Geometry check sheet. Reference: the model listing, model coordinates, mm. A direction names the side the tool comes from. Coordinates: 2 decimals unless noted, no trailing zeros. Write each loop counter-clockwise with the first axis right and the second up, starting at its lowest first coordinate (ties: lowest second). Pieces come first, ordered by that corner, then holes. Notation, with made-up numbers: (56, 15) -> (69, 15) arc R14 cw to (69, 35) -> close; hole circle Ø4 at (24, 22). An arc over 180 degrees is marked (long way). Answer in a Markdown table with one row per item. Add a question column.
1. Cross-section at D-D on z = 7.5. Record the cut outline in (x, y), and give its area (3 significant figures).
2. Cross-section at B-B on x = -2. Record the cut outline in (y, z) (3 decimals).
3. Set-up check for faces 1 (the flat face through (0, 13, 10.033)), 2 (the flat face through (16.05, 12.52, 15.09)), 3 (the flat face through (-12.7, -38, 0)), 4 (the flat face through (0, -38, -3.175)): record each of +Z, -Z, +X, -X, +Y, -Y from which the full face is reachable in a straight line by a thin tool's end or side.
4. Mould release check, pull along Z, two halves, no side actions. Record for faces 5 (the flat face through (-12.954, 13, 7)), 6 (the cylindrical face through (0, 13, -21)), 7 (the cylindrical face through (7.932, -66.542, -0.044)): pulls with the +Z half, pulls with the -Z half, needs draft (parallel to the pull), parting line crosses it, or undercut.
5. Cross-section at A-A on y = -25.4. Record the cut outline in (x, z) (3 decimals).
6. Depth check by flat-ended pin: P1, Ø9, axis at x = -6.35, y = -50.8, coming from the +Z side (3 decimals); P2, Ø7.5, axis at x = 6, y = 17, coming from the -Z side; P3, Ø20.5, axis at x = -1.5, y = -33.5, coming from the -Z side (3 decimals); P4, Ø4, axis at x = -5, z = 3.5, coming from the +Y side. Enter the tip coordinate at first touch or a pass-through.
7. Scan lines: L1, parallel to Y at x = -6.35, z = -1.5; L2, parallel to X at y = -12, z = 0; L3, parallel to X at y = -11.5, z = -2. Record each from-to range of solid material in increasing order. Write a range as from..to.
8. Cross-section at C-C on y = 4.5. Record the cut outline in (x, z) (3 decimals).
```python
from build123d import *

# Parameters (mm, degrees)
BOSS_EXTRUDE1_DEPTH = 25.4
SKETCH3_W           = 25.4
SKETCH3_H           = 69.85
SKETCH3_R           = 3.429
BOSS_EXTRUDE3_DEPTH = 3.175
SKETCH4_W           = 25.908
SKETCH4_H           = 6.858
CUT_EXTRUDE1_DEPTH  = 76.901399855
FILLET2_R           = 5.08


with BuildPart() as part:
    # Sketch1 → Boss-Extrude1 (new body)
    with BuildSketch(Plane(origin=(0, 0, 0), x_dir=(1, 0, 0), z_dir=(0, 1, 0))):
        with BuildLine():
            Line((13.870085237, 15.767711804), (16.343875029, 16.343875029))
            Line((16.343875029, 16.343875029), (15.767711804, 13.870085237))
            ThreePointArc((15.767711804, 13.870085237), (21, 0), (15.767711804, -13.870085237))
            Line((15.767711804, -13.870085237), (16.343875029, -16.343875029))
            Line((16.343875029, -16.343875029), (13.870085237, -15.767711804))
            ThreePointArc((13.870085237, -15.767711804), (0, -21), (-13.870085237, -15.767711804))
            Line((-13.870085237, -15.767711804), (-16.343875029, -16.343875029))
            Line((-16.343875029, -16.343875029), (-15.767711804, -13.870085237))
            ThreePointArc((-15.767711804, -13.870085237), (-21, 0), (-15.767711804, 13.870085237))
            Line((-15.767711804, 13.870085237), (-16.343875029, 16.343875029))
            Line((-16.343875029, 16.343875029), (-13.870085237, 15.767711804))
            ThreePointArc((-13.870085237, 15.767711804), (0, 21), (13.870085237, 15.767711804))
        make_face()
    extrude(amount=BOSS_EXTRUDE1_DEPTH)

    # Sketch3 → Boss-Extrude3 (add, symmetric)
    with BuildSketch(Plane.XY):
        with Locations((0, -34.925)):
            Rectangle(SKETCH3_W, SKETCH3_H)
        with Locations((-6.35, -12.7)):
            Circle(SKETCH3_R, mode=Mode.SUBTRACT)
        with Locations((6.35, -12.7)):
            Circle(SKETCH3_R, mode=Mode.SUBTRACT)
        with Locations((6.35, -25.4)):
            Circle(SKETCH3_R, mode=Mode.SUBTRACT)
        with Locations((6.35, -38.1)):
            Circle(SKETCH3_R, mode=Mode.SUBTRACT)
        with Locations((6.35, -50.8)):
            Circle(SKETCH3_R, mode=Mode.SUBTRACT)
        with Locations((6.35, -63.5)):
            Circle(SKETCH3_R, mode=Mode.SUBTRACT)
        with Locations((-6.35, -25.4)):
            Circle(SKETCH3_R, mode=Mode.SUBTRACT)
        with Locations((-6.35, -38.1)):
            Circle(SKETCH3_R, mode=Mode.SUBTRACT)
        with Locations((-6.35, -50.8)):
            Circle(SKETCH3_R, mode=Mode.SUBTRACT)
        with Locations((-6.35, -63.5)):
            Circle(SKETCH3_R, mode=Mode.SUBTRACT)
    extrude(amount=BOSS_EXTRUDE3_DEPTH, both=True)

    # Sketch4 → Cut-Extrude1 (cut, through all)
    with BuildSketch(Plane(origin=(0, 0, 0), x_dir=(-1, 0, 0), z_dir=(0, -1, 0))):
        with Locations((0, -6.604)):
            Rectangle(SKETCH4_W, SKETCH4_H)
    extrude(amount=-CUT_EXTRUDE1_DEPTH, mode=Mode.SUBTRACT)

    # Fillet2
    # the kernel refuses this fillet: 5.08 mm, written as the material it adds along each edge
    with BuildSketch(Plane(origin=(-12.7, 0, -3.175), x_dir=(-1, 0, 0), z_dir=(0, 0, 1)), Plane(origin=(12.7, 0, 3.175), x_dir=(1, 0, 0), z_dir=(0, 0, -1))) as fillet2_piece_1:
        with BuildLine():
            CenterArc((FILLET2_R, FILLET2_R), FILLET2_R, 180, 90)
            Line((0, FILLET2_R), (-FILLET2_R * 0.02, FILLET2_R))
            Line((-FILLET2_R * 0.02, FILLET2_R), (-FILLET2_R * 0.02, -FILLET2_R * 0.02))
            Line((-FILLET2_R * 0.02, -FILLET2_R * 0.02), (FILLET2_R, -FILLET2_R * 0.02))
            Line((FILLET2_R, -FILLET2_R * 0.02), (FILLET2_R, 0))
        make_face()
    extrude(amount=6.35)
    with BuildSketch(Plane(origin=(-12.7, 0, -3.175), x_dir=(0, 0, -1), z_dir=(1, 0, 0))) as fillet2_piece_2:
        with BuildLine():
            CenterArc((FILLET2_R, -FILLET2_R), FILLET2_R, 90, 90)
            Line((0, -FILLET2_R), (-FILLET2_R * 0.02, -FILLET2_R))
            Line((-FILLET2_R * 0.02, -FILLET2_R), (-FILLET2_R * 0.02, FILLET2_R * 0.02))
            Line((-FILLET2_R * 0.02, FILLET2_R * 0.02), (FILLET2_R, FILLET2_R * 0.02))
            Line((FILLET2_R, FILLET2_R * 0.02), (FILLET2_R, 0))
        make_face()
    extrude(amount=25.4)
    with BuildSketch(Plane(origin=(-25.4, 0, -3.175), x_dir=(0, 0, -1), z_dir=(1, 0, 0))) as fillet2_piece_3a_section:
        with BuildLine():
            CenterArc((FILLET2_R, -FILLET2_R), FILLET2_R, 90, 90)
            Line((0, -FILLET2_R), (-FILLET2_R * 0.02, -FILLET2_R))
            Line((-FILLET2_R * 0.02, -FILLET2_R), (-FILLET2_R * 0.02, FILLET2_R * 0.02))
            Line((-FILLET2_R * 0.02, FILLET2_R * 0.02), (FILLET2_R, FILLET2_R * 0.02))
            Line((FILLET2_R, FILLET2_R * 0.02), (FILLET2_R, 0))
        make_face()
    fillet2_piece_3a = extrude(amount=38.1, mode=Mode.PRIVATE)
    fillet2_piece_3a = split(fillet2_piece_3a, bisect_by=Plane(origin=(-12.7, -1.15008718, -4.32508718), z_dir=(-1, 0, 0)), keep=Keep.TOP, mode=Mode.PRIVATE)
    with BuildSketch(Plane(origin=(-12.7, 0, -15.875), x_dir=(-1, 0, 0), z_dir=(0, 0, 1))) as fillet2_piece_3b_section:
        with BuildLine():
            CenterArc((FILLET2_R, FILLET2_R), FILLET2_R, 180, 90)
            Line((0, FILLET2_R), (-FILLET2_R * 0.02, FILLET2_R))
            Line((-FILLET2_R * 0.02, FILLET2_R), (-FILLET2_R * 0.02, -FILLET2_R * 0.02))
            Line((-FILLET2_R * 0.02, -FILLET2_R * 0.02), (FILLET2_R, -FILLET2_R * 0.02))
            Line((FILLET2_R, -FILLET2_R * 0.02), (FILLET2_R, 0))
        make_face()
    fillet2_piece_3b = extrude(amount=19.05, mode=Mode.PRIVATE)
    fillet2_piece_3b = split(fillet2_piece_3b, bisect_by=Plane(origin=(-13.85008718, -1.15008718, -3.175), z_dir=(0, 0, -1)), keep=Keep.TOP, mode=Mode.PRIVATE)
    fillet2_piece_3 = fillet2_piece_3a & fillet2_piece_3b
    add(fillet2_piece_3)
    with BuildSketch(Plane(origin=(-12.7, 0, -3.175), x_dir=(0, 0, -1), z_dir=(1, 0, 0))) as fillet2_piece_4a_section:
        with BuildLine():
            CenterArc((FILLET2_R, -FILLET2_R), FILLET2_R, 90, 90)
            Line((0, -FILLET2_R), (-FILLET2_R * 0.02, -FILLET2_R))
            Line((-FILLET2_R * 0.02, -FILLET2_R), (-FILLET2_R * 0.02, FILLET2_R * 0.02))
            Line((-FILLET2_R * 0.02, FILLET2_R * 0.02), (FILLET2_R, FILLET2_R * 0.02))
            Line((FILLET2_R, FILLET2_R * 0.02), (FILLET2_R, 0))
        make_face()
    fillet2_piece_4a = extrude(amount=38.1, mode=Mode.PRIVATE)
    fillet2_piece_4a = split(fillet2_piece_4a, bisect_by=Plane(origin=(12.7, -1.15008718, -4.32508718), z_dir=(1, 0, 0)), keep=Keep.TOP, mode=Mode.PRIVATE)
    with BuildSketch(Plane(origin=(12.7, 0, 3.175), x_dir=(1, 0, 0), z_dir=(0, 0, -1))) as fillet2_piece_4b_section:
        with BuildLine():
            CenterArc((FILLET2_R, FILLET2_R), FILLET2_R, 180, 90)
            Line((0, FILLET2_R), (-FILLET2_R * 0.02, FILLET2_R))
            Line((-FILLET2_R * 0.02, FILLET2_R), (-FILLET2_R * 0.02, -FILLET2_R * 0.02))
            Line((-FILLET2_R * 0.02, -FILLET2_R * 0.02), (FILLET2_R, -FILLET2_R * 0.02))
            Line((FILLET2_R, -FILLET2_R * 0.02), (FILLET2_R, 0))
        make_face()
    fillet2_piece_4b = extrude(amount=19.05, mode=Mode.PRIVATE)
    fillet2_piece_4b = split(fillet2_piece_4b, bisect_by=Plane(origin=(13.85008718, -1.15008718, -3.175), z_dir=(0, 0, -1)), keep=Keep.TOP, mode=Mode.PRIVATE)
    fillet2_piece_4 = fillet2_piece_4a & fillet2_piece_4b
    add(fillet2_piece_4)


solid = part.part
```
Results found:
| question | item | result |
|---|---|---|
| 1 | outline | (-19.62, 0) -> (-12.95, 0) -> (-12.95, 25.4) -> (-19.62, 25.4) -> close; (12.95, 0) -> (19.62, 0) -> (19.62, 25.4) -> (12.95, 25.4) -> close |
| 1 | area | 338 mm^2 |
| 2 | outline | (-69.85, -3.175) -> (-5.08, -3.175) arc R5.08 cw to (0, -8.255) -> (0, -20.905) -> (25.4, -20.905) -> (25.4, 3.175) -> (-69.85, 3.175) -> close; (0, 10.033) -> (25.4, 10.033) -> (25.4, 20.905) -> (0, 20.905) -> close |
| 3 | face 1 | +Y, -Y |
| 3 | face 2 | +X, +Y, -Y |
| 3 | face 3 | +Z, -Z, -X, -Y |
| 3 | face 4 | -Z, +X, -X, -Y |
| 4 | face 5 | undercut |
| 4 | face 6 | pulls with the -Z half |
| 4 | face 7 | needs draft |
| 5 | outline | (-12.7, -3.175) -> (-9.779, -3.175) -> (-9.779, 3.175) -> (-12.7, 3.175) -> close; (-2.921, -3.175) -> (2.921, -3.175) -> (2.921, 3.175) -> (-2.921, 3.175) -> close; (9.779, -3.175) -> (12.7, -3.175) -> (12.7, 3.175) -> (9.779, 3.175) -> close |
| 6 | P1 | stops at z = 3.175 |
| 6 | P2 | stops at z = -20.88 |
| 6 | P3 | stops at z = -3.175 |
| 6 | P4 | stops at y = 25.4 |
| 7 | L1 | y = -69.85..-66.93, -60.07..-54.23, -47.37..-41.53, -34.67..-28.83, -21.97..-16.13, -9.27..25.4 |
| 7 | L2 | x = -12.7..-9.71, -2.99..2.99, 9.71..12.7 |
| 7 | L3 | x = -12.7..-9.56, -3.14..3.14, 9.56..12.7 |
| 8 | outline | (-16.344, -16.344) -> (-13.87, -15.768) arc R21 ccw to (13.87, -15.768) -> (16.344, -16.344) -> (15.768, -13.87) arc R21 ccw to (15.768, 13.87) -> (16.344, 16.344) -> (13.87, 15.768) arc R21 ccw to (-13.87, 15.768) -> (-16.344, 16.344) -> (-15.768, 13.87) arc R21 ccw to (-15.768, -13.87) -> close; hole (-12.954, 3.175) -> (12.954, 3.175) -> (12.954, 10.033) -> (-12.954, 10.033) -> close |
